```python
from build123d import *

# Parameters (mm, degrees)
SKETCH2_W           = 29.8
SKETCH2_H           = 25
BOSS_EXTRUDE1_DEPTH = 1.5
SKETCH3_W           = 6.05
SKETCH3_H           = 6.05
BOSS_EXTRUDE2_DEPTH = 3
BOSS_EXTRUDE3_DEPTH = 6.05


with BuildPart() as part:
    # Sketch2 → Boss-Extrude1 (new body)
    with BuildSketch(Plane(origin=(0, 0, 0), x_dir=(0, 1, 0), z_dir=(0, 0, 1))):
        Rectangle(SKETCH2_W, SKETCH2_H)
    extrude(amount=BOSS_EXTRUDE1_DEPTH)

    # Sketch3 → Boss-Extrude2 (add)
    with BuildSketch(Plane.XY.offset(1.5)):
        Rectangle(SKETCH3_W, SKETCH3_H)
    extrude(amount=BOSS_EXTRUDE2_DEPTH)

    # Sketch4 → Boss-Extrude3 (add)
    with BuildSketch(Plane(origin=(0, 3.025, 0), x_dir=(-1, 0, 0), z_dir=(0, 1, 0))):
        Polygon((-3.025, 4.5), (-3.025, 3.7), (-3.225, 3.7), align=None)
        Polygon((3.225, 3.7), (3.025, 4.5), (3.025, 3.7), align=None)
    extrude(amount=-BOSS_EXTRUDE3_DEPTH)


solid = part.part
```
The model under review builds one solid part; all positions refer to its coordinate system, in mm. A direction names the side the tool comes from. Round coordinates to 2 decimals unless told otherwise and drop trailing zeros. Loops run counter-clockwise (first coordinate to the right, second up) from the corner with the lowest first, then second, coordinate; pieces in that order, holes last. Notation, with made-up numbers: (74.5, 53.25) - (93.5, 53.25) arc R17 cw to (93.5, 61.25) - close; hole circle Ø11 at (-7, -27.5). An arc over 180 degrees is marked (long way). Use a Markdown table: item, result. Add a question column.
Q1. Add section D-D (x = 10.5). State the section outline as (y, z) points, plus the area to 3 significant figures.
Q2. Add section B-B (y = 1). State the section outline as (x, z) points (3 decimals).
Q3. Insertion check: pin 1 Ø12 at (x, y) = (-7.5, -3.5) entering from +Z; pin 2 Ø1 at (x, z) = (2, 3) entering from -Y (3 decimals); pin 3 Ø1.1 at (y, z) = (0, 3) entering from -X (3 decimals); pin 4 Ø1 at (x, y) = (2, -7.5) entering from +Z. Each pin has a flat end and moves straight along its axis. Give the tip position at first contact, or say it passes through.
Q4. Add section C-C (z = 2.4). State the section outline as (x, y) points (3 decimals), plus the area to 3 significant figures.
Q5. The part is to be moulded in two halves that separate along Z. For faces 1 (the face through (0, 0, 0)), 2 (the face through (12.5, 0, 1)), 3 (the face through (-3.025, 0, 3)), say which applies: pulls with the +Z half, pulls with the -Z half, needs draft (parallel to the pull), parting line crosses it, or undercut.
Q6. Machinability: for faces 4 (the face through (0, -3.025, 3)), 5 (the face through (3.025, 0, 3)), 6 (the face through (0, 3.025, 3)), which of the approach directions +Z, -Z, +X, -X, +Y, -Y give a long, thin tool a straight path to every point of the face, cutting with its end or side? Answer none if there is none.
Q7. For probe 1 along Z at (x, y) = (3.75, -5.5); probe 2 along Y at (x, z) = (0.75, 2.65) (3 decimals), list the stretches that pass through material, from the lowest coordinate up.
Q8. Add section A-A (x = -2.5). State the section outline as (y, z) points (3 decimals).
Worked answers:
| question | item | result |
|---|---|---|
| 1 | outline | (-14.9, 0) - (14.9, 0) - (14.9, 1.5) - (-14.9, 1.5) - close |
| 1 | area | 44.7 mm² |
| 2 | outline | (-12.5, 0) - (12.5, 0) - (12.5, 1.5) - (3.025, 1.5) - (3.025, 3.7) - (3.225, 3.7) - (3.025, 4.5) - (-3.025, 4.5) - (-3.225, 3.7) - (-3.025, 3.7) - (-3.025, 1.5) - (-12.5, 1.5) - close |
| 3 | pin 1 | z = 4.5 |
| 3 | pin 2 | y = -3.025 |
| 3 | pin 3 | x = -3.025 |
| 3 | pin 4 | z = 1.5 |
| 4 | outline | (-3.025, -3.025) - (3.025, -3.025) - (3.025, 3.025) - (-3.025, 3.025) - close |
| 4 | area | 36.6 mm² |
| 5 | face 1 | pulls with the -Z half |
| 5 | face 2 | needs draft |
| 5 | face 3 | undercut |
| 6 | face 4 | +Z, +X, -X, -Y |
| 6 | face 5 | +X, +Y, -Y |
| 6 | face 6 | +Z, +X, -X, +Y |
| 7 | probe 1 | 0 to 1.5 |
| 7 | probe 2 | -3.025 to 3.025 |
| 8 | outline | (-14.9, 0) - (14.9, 0) - (14.9, 1.5) - (3.025, 1.5) - (3.025, 4.5) - (-3.025, 4.5) - (-3.025, 1.5) - (-14.9, 1.5) - close |
